```python
from build123d import *

# Parameters (mm, degrees)
F1_DEPTH = 1.2


with BuildPart() as f1:
    # F0 (on Top) → F1 (new body)
    with BuildSketch(Plane.XY):
        with BuildLine():
            ThreePointArc((-11.057271, 14.742629), (-11.634473, 15.191614), (-11.432224, 15.894354))
            ThreePointArc((-11.432224, 15.894354), (-10.153228, 20.506336), (-14.117182, 23.188365))
            ThreePointArc((-14.117182, 23.188365), (-36.512956, 0.2125), (-14.246818, -22.88902))
            ThreePointArc((-14.246818, -22.88902), (-11.548187, -21.994576), (-10.080089, -19.559965))
            ThreePointArc((-10.080089, -19.559965), (-10.072004, -19.503727), (-10.060345, -19.448119))
            ThreePointArc((-10.060345, -19.448119), (-9.547743, -18.841405), (-8.754742, -18.886272))
            ThreePointArc((-8.754742, -18.886272), (-8.700528, -18.919907), (-8.648865, -18.957342))
            ThreePointArc((-8.648865, -18.957342), (-6.352939, -19.617532), (-4.078768, -18.885911))
            ThreePointArc((-4.078768, -18.885911), (-0.715713, -18.386761), (1.721045, -20.75773))
            ThreePointArc((1.721045, -20.75773), (5.586952, -23.492169), (9.452858, -20.75773))
            ThreePointArc((9.452858, -20.75773), (11.889616, -18.386761), (15.252671, -18.885911))
            ThreePointArc((15.252671, -18.885911), (17.843085, -19.610271), (20.324967, -18.573352))
            ThreePointArc((20.324967, -18.573352), (20.860199, -18.525989), (21.184551, -18.954373))
            ThreePointArc((21.184551, -18.954373), (21.18943, -19.004364), (21.189767, -19.054592))
            ThreePointArc((21.189767, -19.054592), (22.528031, -21.829393), (25.420721, -22.88902))
            ThreePointArc((25.420721, -22.88902), (47.686792, 0.062182), (25.591536, 23.177874))
            ThreePointArc((25.591536, 23.177874), (21.499758, 20.276401), (23.278403, 15.586239))
            ThreePointArc((23.278403, 15.586239), (23.467753, 14.985609), (22.973846, 14.594884))
            ThreePointArc((22.973846, 14.594884), (22.937343, 14.593682), (22.90084, 14.594884))
            Line((22.90084, 14.594884), (17.09098, 14.594884))
            Line((17.09098, 14.594884), (14.143941, 21.317934))
            ThreePointArc((14.143941, 21.317934), (10.606114, 23.766142), (6.829072, 21.706071))
            Line((6.829072, 21.706071), (6.364495, 20.893062))
            Line((6.364495, 20.893062), (5.454447, 20.917279))
            Line((5.454447, 20.917279), (4.919283, 21.853817))
            ThreePointArc((4.919283, 21.853817), (1.142241, 23.913887), (-2.395586, 21.465679))
            Line((-2.395586, 21.465679), (-5.342625, 14.742629))
            Line((-5.342625, 14.742629), (-10.971048, 14.742629))
            ThreePointArc((-10.971048, 14.742629), (-11.01416, 14.741203), (-11.057271, 14.742629))
        make_face()
        with BuildLine():
            ThreePointArc((-14.110806, -18.891334), (-32.512973, 0.201246), (-14.003666, 19.189977))
            ThreePointArc((-14.003666, 19.189977), (-13.903576, 19.113297), (-13.958097, 18.999607))
            ThreePointArc((-13.958097, 18.999607), (-16.427445, 14.482007), (-12.888596, 10.74263))
            Line((-12.888596, 10.74263), (-2.728596, 10.74263))
            Line((-2.728596, 10.74263), (1.2679, 19.859795))
            ThreePointArc((1.2679, 19.859795), (1.354189, 19.919508), (1.446312, 19.869262))
            Line((1.446312, 19.869262), (3.098136, 16.978568))
            Line((3.098136, 16.978568), (8.650219, 16.830822))
            Line((8.650219, 16.830822), (10.302044, 19.721517))
            ThreePointArc((10.302044, 19.721517), (10.394167, 19.771763), (10.480455, 19.71205))
            Line((10.480455, 19.71205), (14.476952, 10.594885))
            Line((14.476952, 10.594885), (24.636952, 10.594885))
            ThreePointArc((24.636952, 10.594885), (28.19471, 14.507176), (25.386326, 18.987873))
            ThreePointArc((25.386326, 18.987873), (25.323767, 19.101427), (25.425881, 19.181307))
            ThreePointArc((25.425881, 19.181307), (43.686821, 0.077013), (25.284709, -18.891334))
            ThreePointArc((25.284709, -18.891334), (25.183808, -18.813608), (25.241076, -18.699842))
            ThreePointArc((25.241076, -18.699842), (27.330713, -15.158302), (24.636952, -12.051417))
            ThreePointArc((24.636952, -12.051417), (20.65623, -12.820988), (17.676245, -15.570182))
            ThreePointArc((17.676245, -15.570182), (17.611536, -15.615886), (17.533888, -15.600178))
            ThreePointArc((17.533888, -15.600178), (10.661063, -14.580103), (5.681242, -19.425476))
            ThreePointArc((5.681242, -19.425476), (5.586952, -19.49217), (5.492661, -19.425476))
            ThreePointArc((5.492661, -19.425476), (0.51284, -14.580103), (-6.359985, -15.600178))
            ThreePointArc((-6.359985, -15.600178), (-6.437633, -15.615886), (-6.502342, -15.570182))
            ThreePointArc((-6.502342, -15.570182), (-9.482327, -12.820988), (-13.463048, -12.051417))
            ThreePointArc((-13.463048, -12.051417), (-16.15681, -15.158302), (-14.067173, -18.699842))
            ThreePointArc((-14.067173, -18.699842), (-14.009905, -18.813608), (-14.110806, -18.891334))
        make_face(mode=Mode.SUBTRACT)
        with BuildLine():
            Line((-10.971048, 14.742629), (-11.057271, 14.742629))
            ThreePointArc((-11.057271, 14.742629), (-11.01416, 14.741203), (-10.971048, 14.742629))
        make_face()
        with BuildLine():
            ThreePointArc((-10.060345, -19.448119), (-10.072004, -19.503727), (-10.080089, -19.559965))
            ThreePointArc((-10.080089, -19.559965), (-10.06983, -19.50411), (-10.060345, -19.448119))
        make_face()
        with BuildLine():
            ThreePointArc((-8.648865, -18.957342), (-8.700528, -18.919907), (-8.754742, -18.886272))
            ThreePointArc((-8.754742, -18.886272), (-8.702079, -18.922219), (-8.648865, -18.957342))
        make_face()
        with BuildLine():
            Line((22.973846, 14.594884), (22.90084, 14.594884))
            ThreePointArc((22.90084, 14.594884), (22.937343, 14.593682), (22.973846, 14.594884))
        make_face()
        with BuildLine():
            ThreePointArc((21.189767, -19.054592), (21.18943, -19.004364), (21.184551, -18.954373))
            ThreePointArc((21.184551, -18.954373), (21.186852, -19.004498), (21.189767, -19.054592))
        make_face()
    extrude(amount=F1_DEPTH)


solid = f1.part
```
Work out the finished part from the listing and answer in its coordinate system (mm). A direction names the side the tool comes from. Coordinates: 2 decimals unless noted, no trailing zeros. Order: outer loops, then holes, each group sorted by start corner. A loop starts at its lowest first (then second) coordinate and runs counter-clockwise, first axis right, second up. Notation, with made-up numbers: M 36.25,89 L 42.25,89 A21 ccw 42.25,93 Z; hole C 23,-33.5 d7. An arc over 180 degrees is marked long. Use CSV: the item, a comma, the result in double quotes.
1) Consider line 1 (X direction, y = -19, z = 0.85); line 2 (X direction, y = 11.5, z = 0.8); line 3 (X direction, y = 5, z = 1.05). Determine where each line is inside the solid, lowest interval first. Write a range as [from, to].
Worked out:
line 1,"x = [-26.3, -9.79], [-8.58, -4.25], [0.45, 5.33], [5.85, 10.73], [15.43, 19.76], [21.19, 37.47]"
line 2,"x = [-33.52, -28.76], [-14.65, -2.4], [14.08, 26.6], [39.93, 44.7]"
line 3,"x = [-36, -31.88], [43.06, 47.17]"
2) Determine the mould class of faces 1 (the face through (1.206, 23.917, 0.592)), 2 (the face through (11.843, -18.402, 0.592)), 3 (the face through (10.76, -14.55, 0.59)), 4 (the face through (-16.15, -15.1, 0.59)) for opening direction Y: released by +Y, released by -Y, zero draft, split by the parting line, or undercut.
Worked out:
face 1,"released by +Y"
face 2,"released by -Y"
face 3,"undercut"
face 4,"undercut"
3) A flat-ended cylindrical pin translates along its axis: pin 1 Ø0.6 at (x, z) = (19, 1) entering from +Y. Find the tip coordinate at first contact, or state that the pin passes through.
Worked out:
pin 1,"stops at y = 14.59"
4) Section B-B on y = -8.5 is taken. Write down the section's boundary in (x, z), plus the area to 3 significant figures.
Worked out:
outline,"M -34.83,0 L -30.44,0 L -30.44,1.2 L -34.83,1.2 Z; M 41.61,0 L 46,0 L 46,1.2 L 41.61,1.2 Z"
area,"10.5 mm^2"
5) Section A-A on x = -22.5 is taken. Write down the section's boundary in (y, z).
Worked out:
outline,"M -21.06,0 L -16.62,0 L -16.62,1.2 L -21.06,1.2 Z; M 16.92,0 L 21.35,0 L 21.35,1.2 L 16.92,1.2 Z"
6) For faces 5 (the face through (15.638, 17.909, 0.592)), 6 (the face through (15, 11, 0)), 7 (the face through (22.495, -21.8, 0.592)), 8 (the face through (-32.51, -0.21, 0.59)), 9 (the face through (15, 11, 1.2)), determine the directions among +Z, -Z, +X, -X, +Y, -Y from which every point of the face is accessible in a straight line to the end or side of a thin tool.
Worked out:
face 5,"+Z, -Z, +Y"
face 6,"-Z, +X, -X, +Y, -Y"
face 7,"+Z, -Z, -Y"
face 8,"+Z, -Z"
face 9,"+Z, +X, -X, +Y, -Y"
